Build history of the part. All positions in model axes, mm. Face numbers are marked on the shaded views. A direction names the side the tool comes from. Round coordinates to 2 decimals unless told otherwise and drop trailing zeros. Write each loop counter-clockwise with the first axis right and the second up, starting at its lowest first coordinate (ties: lowest second). Pieces come first, ordered by that corner, then holes. Notation, with made-up numbers: (1.25, 11.25) - (24.25, 11.25) arc R5 ccw to (24.25, 15.25) - close; hole circle Ø9 at (-5, -36.5). An arc over 180 degrees is marked (long way). Write each question's results on one line, items separated by ' | '.
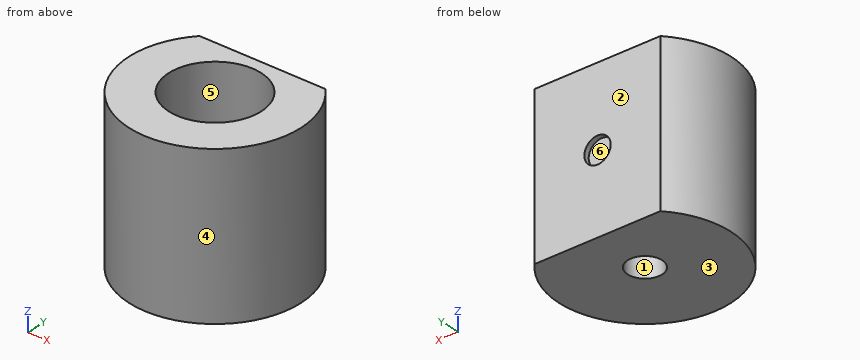
from build123d import *

# Parameters (mm, degrees)
SKETCH1_R           = 32.5
BOSS_EXTRUDE1_DEPTH = 60
SKETCH3_R           = 17.5
CUT_EXTRUDE4_DEPTH  = 52
SKETCH6_R           = 6.5
CUT_EXTRUDE5_DEPTH  = 8
SKETCH8_W           = 65.355871795
SKETCH8_H           = 11.921493712
CUT_EXTRUDE6_DEPTH  = 60
SKETCH9_R           = 5
CUT_EXTRUDE9_DEPTH  = 2


with BuildPart() as part:
    # Sketch1 → Boss-Extrude1 (new body)
    with BuildSketch(Plane.XY):
        Circle(SKETCH1_R)
    extrude(amount=BOSS_EXTRUDE1_DEPTH)

    # Sketch3 → Cut-Extrude4 (cut)
    with BuildSketch(Plane.XY.offset(60)):
        Circle(SKETCH3_R)
    extrude(amount=-CUT_EXTRUDE4_DEPTH, mode=Mode.SUBTRACT)

    # Sketch6 → Cut-Extrude5 (cut)
    with BuildSketch(Plane.XY.offset(8)):
        Circle(SKETCH6_R)
    extrude(amount=-CUT_EXTRUDE5_DEPTH, mode=Mode.SUBTRACT)

    # Sketch8 → Cut-Extrude6 (cut)
    with BuildSketch(Plane.XY.offset(60)):
        with Locations((-1.31264436, 27.960746856)):
            Rectangle(SKETCH8_W, SKETCH8_H)
    extrude(amount=-CUT_EXTRUDE6_DEPTH, mode=Mode.SUBTRACT)

    # Sketch9 → Cut-Extrude9 (cut)
    with BuildSketch(Plane(origin=(0, 22, 0), x_dir=(1, 0, 0), z_dir=(0, 1, 0))):
        with Locations(Location((0, -30, 0), (0, 0, 270))):  # turned: the seam where the file's is
            Circle(SKETCH9_R)
    extrude(amount=-CUT_EXTRUDE9_DEPTH, mode=Mode.SUBTRACT)


solid = part.part
(1) Two-plate mould, pull along Y, no slides. Class the marked faces 1, 2 and 3: released by +Y, released by -Y, zero draft, split by the parting line, or undercut.
Worked answers:
face 1: undercut | face 2: released by +Y | face 3: zero draft
(2) Drill centre lines: probe 1 along Y at (x, z) = (0, 4.25); probe 2 along Z at (x, y) = (-4.5, 11); probe 3 along Y at (x, z) = (-14, 27.5). Where is each one in solid material? Low to high. Write a range as [from, to].
Worked answers:
probe 1: y = [-32.5, -6.5], [6.5, 22] | probe 2: z = [0, 8] | probe 3: y = [-29.33, -10.5], [10.5, 22]
(3) Slice it at B-B, the plane x = 0. Write the cut outline in (y, z), and give its area (3 significant figures).
Worked answers:
outline: (-32.5, 0) - (-6.5, 0) - (-6.5, 8) - (-17.5, 8) - (-17.5, 60) - (-32.5, 60) - close; (6.5, 0) - (22, 0) - (22, 25) - (20, 25) - (20, 35) - (22, 35) - (22, 60) - (17.5, 60) - (17.5, 8) - (6.5, 8) - close | area: 1,330 mm2
(4) Flat gauge pins, fed straight in: pin 1 Ø5 at (x, z) = (7, 12) entering from -Y; pin 2 Ø2 at (y, z) = (1.5, 52.5) entering from +X; pin 3 Ø4 at (y, z) = (10.5, 37) entering from -X. Where does each tip first touch, or does it go through?
Worked answers:
pin 1: stops at y = -32.19 | pin 2: stops at x = 32.5 | pin 3: stops at x = -31.37
(5) Tool access for the marked faces 4, 5 and 6: list every direction of +Z, -Z, +X, -X, +Y, -Y with a clear straight run to the whole face (end or side of a thin tool).
Worked answers:
face 4: +Z, -Z | face 5: +Z | face 6: +Y
(6) Slice it at D-D, the plane y = 8.5. Write the cut outline in (x, z), and give its area (3 significant figures).
Worked answers:
outline: (-31.37, 0) - (31.37, 0) - (31.37, 60) - (15.3, 60) - (15.3, 8) - (-15.3, 8) - (-15.3, 60) - (-31.37, 60) - close | area: 2,170 mm2
(7) Slice it at C-C, the plane z = 6.5. Write the cut outline in (x, y).
Worked answers:
outline: (-23.92, 22) arc R32.5 ccw (long way) to (23.92, 22) - close; hole circle Ø13 at (0, 0)
(8) Slice it at A-A, the plane y = 0. Write the cut outline in (x, z).
Worked answers:
outline: (-32.5, 0) - (-6.5, 0) - (-6.5, 8) - (-17.5, 8) - (-17.5, 60) - (-32.5, 60) - close; (6.5, 0) - (32.5, 0) - (32.5, 60) - (17.5, 60) - (17.5, 8) - (6.5, 8) - close
